from build123d import *

# Parameters (mm, degrees)
SKETCH1_R              = 47
BASE_EXTRUDE_DEPTH     = 6.35
M8_CLEARANCE_HOLES_D   = 9
CIRPATTERN_COUNT       = 6
CUT_EXTRUDE_DEPTH      = 67.770670957
CUT_EXTRUDE_DEPTH_BACK = 67.770670957
CHAMFER1_SIZE          = 0.635
SKETCH8_R              = 12.7
SHAFT_EXTRUDE_DEPTH    = 51.76000062
CHAMFER3_SIZE          = 0.635
SHAFT_CHAMFER_SIZE     = 1
SKETCH30_R             = 27.89936
SKETCH30_R_2           = 24.72436
LIP_EXTRUDE_DEPTH      = 5.99948
LIP_CHAMFER_SIZE       = 1.27
CUT_EXTRUDE1_START     = -15
SKETCH45_R             = 12.7
SKETCH45_R_2           = 8.5
CUT_EXTRUDE1_DEPTH     = 15
CHAMFER4_SIZE          = 0.635
FILLET2_R              = 2.54
CUT_EXTRUDE3_DEPTH     = 3.175
FILLET3_R              = 2.54


with BuildPart() as part:
    # Sketch1 → Base-Extrude (new body)
    with BuildSketch(Plane(origin=(0, 0, 0), x_dir=(0, 0, -1), z_dir=(1, 0, 0))):
        Circle(SKETCH1_R)
    extrude(amount=-BASE_EXTRUDE_DEPTH)

    # M8 Clearance Holes (through all)
    with Locations(Plane(origin=(0, 0, 0), x_dir=(0, 0, -1), z_dir=(1, 0, 0))):
        with Locations((0, -37.5)):
            m8_clearance_holes = Hole(M8_CLEARANCE_HOLES_D / 2)

    # CirPattern: M8 Clearance Holes ×6 about axis
    cirpattern_axis = Axis((0, 0, 0), (1, 0, 0))
    for i in range(1, CIRPATTERN_COUNT):
        add(m8_clearance_holes.rotate(cirpattern_axis, i * 360 / CIRPATTERN_COUNT), mode=Mode.SUBTRACT)

    # Sketch19 → Cut-Extrude (cut, two sides: drawn at the far end of the back side and taken through both)
    with BuildSketch(Plane(origin=(0, 0, 0), x_dir=(0, 0, -1), z_dir=(1, 0, 0)).offset(-CUT_EXTRUDE_DEPTH_BACK)):
        with BuildLine():
            ThreePointArc((9.274838239, 35.443941724), (14.114033661, 24.446223401), (26.057934823, 25.754216393))
            ThreePointArc((26.057934823, 25.754216393), (33.921184851, 28.139425108), (40.703194264, 23.499999504))
            ThreePointArc((40.703194264, 23.499999504), (23.500000227, 40.703193847), (-4.7e-08, 47))
            ThreePointArc((-4.7e-08, 47), (7.40886473, 43.446320157), (9.274838239, 35.443941724))
        make_face()
        with BuildLine():
            ThreePointArc((-26.057934823, 25.754216393), (-14.114033661, 24.446223401), (-9.274838239, 35.443941724))
            ThreePointArc((-9.274838239, 35.443941724), (-7.40886476, 43.44632012), (-4.7e-08, 47))
            ThreePointArc((-4.7e-08, 47), (-23.500000787, 40.703193523), (-40.703194863, 23.499998466))
            ThreePointArc((-40.703194863, 23.499998466), (-33.921185443, 28.139425017), (-26.057934823, 25.754216393))
        make_face()
        with BuildLine():
            ThreePointArc((40.703193464, -23.50000089), (47, -8e-07), (40.703194264, 23.499999504))
            ThreePointArc((40.703194264, 23.499999504), (41.33004921, 15.30689472), (35.332773062, 9.689725331))
            ThreePointArc((35.332773062, 9.689725331), (28.228067323, 0), (35.332773062, -9.689725331))
            ThreePointArc((35.332773062, -9.689725331), (41.330049499, -15.306895465), (40.703193464, -23.50000089))
        make_face()
        with BuildLine():
            ThreePointArc((-35.332773062, 9.689725331), (-41.330048992, 15.306894161), (-40.703194863, 23.499998466))
            ThreePointArc((-40.703194863, 23.499998466), (-47, -6.9e-08), (-40.703194794, -23.499998586))
            ThreePointArc((-40.703194794, -23.499998586), (-41.330049018, -15.306894226), (-35.332773062, -9.689725331))
            ThreePointArc((-35.332773062, -9.689725331), (-28.228067323, 0), (-35.332773062, 9.689725331))
        make_face()
        with BuildLine():
            ThreePointArc((-26.057934823, -25.754216393), (-33.921185375, -28.139425028), (-40.703194794, -23.499998586))
            ThreePointArc((-40.703194794, -23.499998586), (-23.500000688, -40.703193581), (4.4e-08, -47))
            ThreePointArc((4.4e-08, -47), (-7.408864732, -43.446320155), (-9.274838239, -35.443941724))
            ThreePointArc((-9.274838239, -35.443941724), (-14.114033661, -24.446223401), (-26.057934823, -25.754216393))
        make_face()
        with BuildLine():
            ThreePointArc((4.4e-08, -47), (23.499999574, -40.703194224), (40.703193464, -23.50000089))
            ThreePointArc((40.703193464, -23.50000089), (33.92118406, -28.13942523), (26.057934823, -25.754216393))
            ThreePointArc((26.057934823, -25.754216393), (14.114033661, -24.446223401), (9.274838239, -35.443941724))
            ThreePointArc((9.274838239, -35.443941724), (7.408864759, -43.446320121), (4.4e-08, -47))
        make_face()
    extrude(amount=CUT_EXTRUDE_DEPTH + CUT_EXTRUDE_DEPTH_BACK, mode=Mode.SUBTRACT)

    # Chamfer1
    chamfer1_edges = [part.edges().sort_by_distance(p)[0] for p in [
        (-6.35, -24.446223401, 14.114033661),
        (-6.35, 24.446223401, -14.114033661),
        (-6.35, 24.446223401, 14.114033661),
        (-6.35, 23.5, 40.703193978),
        (-6.35, 47, 0),
        (-6.35, -24.446223401, -14.114033661),
        (-6.35, -23.5, -40.703193978),
        (-6.35, -47, 0),
        (-6.35, 0, 28.228067323),
        (-6.35, -23.5, 40.703193978),
        (-6.35, 0, -28.228067323),
        (-6.35, 23.5, -40.703193978),
    ]]
    chamfer(chamfer1_edges, length=CHAMFER1_SIZE)

    # Sketch8 → Shaft-Extrude (add)
    with BuildSketch(Plane.ZY.offset(6.35)):
        with Locations(Location((0, 0, 0), (0, 0, 180))):
            Circle(SKETCH8_R)
    extrude(amount=SHAFT_EXTRUDE_DEPTH)

    # Chamfer3
    chamfer3_edges = [part.edges().sort_by_distance(p)[0] for p in [
        (0, 24.446223401, -14.114033661),
        (0, -24.446223401, 14.114033661),
        (0, -24.446223401, -14.114033661),
        (0, -47, 0),
        (0, -23.5, -40.703193978),
        (0, 24.446223401, 14.114033661),
        (0, 47, 0),
        (0, 23.5, 40.703193978),
        (0, 0, -28.228067323),
        (0, 23.5, -40.703193978),
        (0, 0, 28.228067323),
        (0, -23.5, 40.703193978),
    ]]
    chamfer(chamfer3_edges, length=CHAMFER3_SIZE)

    # Shaft Chamfer
    shaft_chamfer_edges = [part.edges().sort_by_distance(p)[0] for p in [
        (-58.11000062, 0, 12.7),
    ]]
    chamfer(shaft_chamfer_edges, length=SHAFT_CHAMFER_SIZE)

    # Sketch30 → Lip Extrude (add)
    with BuildSketch(Plane(origin=(0, 0, 0), x_dir=(0, 0, -1), z_dir=(1, 0, 0))):
        with Locations(Location((0, 0, 0), (0, 0, 175.528743947))):
            Circle(SKETCH30_R)
        with Locations(Location((0, 0, 0), (0, 0, 180))):
            Circle(SKETCH30_R_2, mode=Mode.SUBTRACT)
    extrude(amount=LIP_EXTRUDE_DEPTH)

    # Lip Chamfer
    lip_chamfer_edges = [part.edges().sort_by_distance(p)[0] for p in [
        (5.99948, 0, -24.72436),
    ]]
    chamfer(lip_chamfer_edges, length=LIP_CHAMFER_SIZE)

    # Sketch45 → Cut-Extrude1 (cut)
    with BuildSketch(Plane.ZY.offset(58.11000062).offset(CUT_EXTRUDE1_START)):
        with Locations(Location((0, 0, 0), (0, 0, 180))):
            Circle(SKETCH45_R)
        Circle(SKETCH45_R_2, mode=Mode.SUBTRACT)
    extrude(amount=CUT_EXTRUDE1_DEPTH, mode=Mode.SUBTRACT)

    # Chamfer4
    chamfer4_edges = [part.edges().sort_by_distance(p)[0] for p in [
        (-43.11000062, 0, 12.7),
    ]]
    chamfer(chamfer4_edges, length=CHAMFER4_SIZE)

    # Fillet2
    fillet2_edges = [part.edges().sort_by_distance(p)[0] for p in [
        (-6.35, 0, 12.7),
    ]]
    fillet(fillet2_edges, radius=FILLET2_R)

    # Sketch48 → Cut-Extrude3 (cut)
    with BuildSketch(Plane.XY.offset(12.7)):
        with BuildLine():
            ThreePointArc((-19.61500062, 0), (-20.54493659, 2.24506403), (-22.79000062, 3.175))
            Line((-22.79000062, 3.175), (-43.11000062, 3.175))
            Line((-43.11000062, 3.175), (-43.11000062, 0))
            Line((-43.11000062, 0), (-19.61500062, 0))
        make_face()
        with BuildLine():
            ThreePointArc((-22.79000062, -3.175), (-20.54493659, -2.24506403), (-19.61500062, 0))
            Line((-19.61500062, 0), (-43.11000062, 0))
            Line((-43.11000062, 0), (-43.11000062, -3.175))
            Line((-43.11000062, -3.175), (-22.79000062, -3.175))
        make_face()
    extrude(amount=-CUT_EXTRUDE3_DEPTH, mode=Mode.SUBTRACT)

    # Fillet3
    # the kernel refuses this fillet: 2.54 mm, written as the material it adds along each edge
    with BuildSketch(Plane(origin=(-43.11000062, 0, 0), x_dir=(0, 0, 1), z_dir=(0, -1, 0))) as fillet3_piece_1_section:
        with BuildLine():
            CenterArc((8.5 + FILLET3_R, FILLET3_R), FILLET3_R, 180, 90)
            Line((8.5, FILLET3_R), (8.5, 0))
            Line((8.5, 0), (8.5 + FILLET3_R, 0))
        make_face()
    fillet3_piece_1 = revolve(axis=Axis((-43.11000062, 0, 0), (-1, 0, 0)), mode=Mode.PRIVATE)
    fillet3_piece_1 = split(fillet3_piece_1, bisect_by=Plane(origin=(-43.740743276, 3.41e-07, 9.525), z_dir=(0, 0, -1)), keep=Keep.TOP, mode=Mode.PRIVATE)
    add(fillet3_piece_1)
    with BuildSketch(Plane(origin=(-43.11000062, 0, 0), x_dir=(0, 0, 1), z_dir=(0, -1, 0))) as fillet3_piece_2_section:
        with BuildLine():
            CenterArc((8.5 + FILLET3_R, FILLET3_R), FILLET3_R, 180, 90)
            Line((8.5, FILLET3_R), (8.5, 0))
            Line((8.5, 0), (8.5 + FILLET3_R, 0))
        make_face()
    fillet3_piece_2 = revolve(axis=Axis((-43.11000062, 0, 0), (-1, 0, 0)), mode=Mode.PRIVATE)
    fillet3_piece_2 = split(fillet3_piece_2, bisect_by=Plane(origin=(-43.151597018, 3.175, 9.740498965), z_dir=(0, 1, 0)), keep=Keep.TOP, mode=Mode.PRIVATE)
    add(fillet3_piece_2)
    with BuildSketch(Plane(origin=(-43.11000062, 0, 0), x_dir=(0, 0, 1), z_dir=(0, -1, 0))) as fillet3_piece_3_section:
        with BuildLine():
            CenterArc((8.5 + FILLET3_R, FILLET3_R), FILLET3_R, 180, 90)
            Line((8.5, FILLET3_R), (8.5, 0))
            Line((8.5, 0), (8.5 + FILLET3_R, 0))
        make_face()
    fillet3_piece_3 = revolve(axis=Axis((-43.11000062, 0, 0), (-1, 0, 0)), mode=Mode.PRIVATE)
    fillet3_piece_3 = split(fillet3_piece_3, bisect_by=Plane(origin=(-43.151597018, -3.175, 9.740498965), z_dir=(0, -1, 0)), keep=Keep.TOP, mode=Mode.PRIVATE)
    add(fillet3_piece_3)


solid = part.part
The listing builds one solid part. Answer for the finished solid, in the listing's coordinates (mm). A direction names the side the tool comes from. Round coordinates to 2 decimals unless told otherwise and drop trailing zeros. Write each loop counter-clockwise with the first axis right and the second up, starting at its lowest first coordinate (ties: lowest second). Pieces come first, ordered by that corner, then holes. Notation, with made-up numbers: (51, 36) - (90, 36) arc R35 cw to (90, 73) - close; hole circle Ø11 at (80, -11.75). An arc over 180 degrees is marked (long way). Use a Markdown table: item, result. Add a question column.
1. Consider line 1 (Z direction, x = -1, y = 18); line 2 (X direction, y = 19.5, z = 27); line 3 (X direction, y = 26, z = -1). Determine where each line is inside the solid, lowest interval first.
2. For a pull along Y with two mould halves and no side action, classify faces 5 (the face through (-25.447, -3.815, -12.114)), 6 (the face through (0, 0, 0)), 7 (the face through (0, -15, -28)) as +Y half, -Y half, draft (parallel to the pull), parting line (faces both ways), or undercut.
3. Flat-ended cylindrical pins translate along their axes: P1, Ø12, axis at x = -6.5, y = -12, coming from the +Z side; P2, Ø4, axis at x = -37.5, y = -5.5, coming from the -Z side; P3, Ø3, axis at x = -4.5, y = 31.5, coming from the +Z side; P4, Ø5.5, axis at y = -18.75, z = -32.48, coming from the -X side. Find the tip coordinate at first contact, or state that the pin passes through.
4. A tool of negligible diameter and unlimited length cuts with its end or side. For faces 1 (the face through (-31, 0, 9.525)), 2 (the face through (2.958, 26.682, -8.153)), 3 (the face through (-3.22, -41.89, -0.98)), 4 (the face through (-51.793, 7.167, 4.57)), from which of +Z, -Z, +X, -X, +Y, -Y can it reach the whole face along a straight path? Write none if from no direction.
5. The part is cut by section C-C (z = 2). Give the number of separate pieces and of enclosed holes in the cut face, and give its area (3 significant figures).
6. The part is cut by section B-B (x = -11.5). Write down the section's boundary in (y, z), and give its area (3 significant figures).
7. The part is cut by section A-A (y = -37.5). Write down the section's boundary in (x, z) (3 decimals), and give its area (3 significant figures).
Reported:
| question | item | result |
|---|---|---|
| 1 | line 1 | -41.95 to -36.91, -28.04 to 28.04, 36.91 to 41.95 |
| 1 | line 2 | -6.35 to 0 |
| 1 | line 3 | -6.35 to 6 |
| 2 | face 5 | parting line |
| 2 | face 6 | undercut |
| 2 | face 7 | draft |
| 3 | P1 | z = 41.94 |
| 3 | P2 | z = -12.21 |
| 3 | P3 | z = 9.57 |
| 3 | P4 | through |
| 4 | face 1 | +Z, -X |
| 4 | face 2 | +X |
| 4 | face 3 | +X, -X |
| 4 | face 4 | -X |
| 5 | separate pieces | 3 |
| 5 | enclosed holes | 0 |
| 5 | area | 1,700 mm^2 |
| 6 | outline | circle Ø25.4 at (0, 0) |
| 6 | area | 507 mm^2 |
| 7 | outline | (-6.35, -8.865) - (-5.715, -9.5) - (-0.635, -9.5) - (0, -8.865) - (0, -4.5) - (-6.35, -4.5) - close; (-6.35, 4.5) - (0, 4.5) - (0, 8.865) - (-0.635, 9.5) - (-5.715, 9.5) - (-6.35, 8.865) - close |
| 7 | area | 62.7 mm^2 |
